Geometry: final body of the model. Coordinates: model frame, mm. A direction names the side the tool comes from. Give positions to 0.01 mm unless a question says otherwise; leave off trailing zeros. Write each loop counter-clockwise with the first axis right and the second up, starting at its lowest first coordinate (ties: lowest second). Pieces come first, ordered by that corner, then holes. Notation, with made-up numbers: (9.5, 86.5) - (27.5, 86.5) arc R19 cw to (27.5, 122.5) - close; hole circle Ø1 at (-33, 45). An arc over 180 degrees is marked (long way). Use CSV: the item, a comma, the result in double quotes. Start each with the question number.
(1) First-contact query: pin 1 Ø4 at (x, y) = (0, 0) entering from +Z. Flat tip, straight axial feed; report the tip coordinate or a pass-through.
(2) Section A-A on z = 3.75. Output: boundary loops of the cut face in (x, y).
(3) Draft query along X for faces 3 (the flat face through (0, 10, 6)), 4 (the flat face through (-10, 0, 6)), 5 (the flat face through (3, 0, 7)), 6 (the cylindrical face through (9.715, 9.699, 6.591)). Return one class per face: released by +X, released by -X, zero draft, split by the parting line, or undercut.
(4) Line query: probe 1 along Y at (x, z) = (0, 5.4); probe 2 along Y at (x, z) = (0, 2); probe 3 along Z at (x, y) = (-3.75, -6.25). Output: solid intervals per line, ascending. Write a range as [from, to].
(5) Section C-C on y = -0.75. Output: boundary loops of the cut face in (x, z).
(6) Section B-B on x = 0. Output: boundary loops of the cut face in (y, z).
(7) Section D-D on z = 7.5. Output: boundary loops of the cut face in (x, y), and give its area (3 significant figures).
(8) Reachability of faces 1 (the flat face through (0, -10, 6)), 2 (the flat face through (-5, 0, 10)) from +Z, -Z, +X, -X, +Y, -Y: full face, straight path, thin tool, end or side. Return the list, or none.
from build123d import *

# Parameters (mm, degrees)
F0_W      = 20
F0_H      = 20
F1_DEPTH  = 13
F2_R      = 1
F3_W      = 10
F3_H      = 11.2
F4_DEPTH  = 6
F5_R      = 2.75
F6_DEPTH  = 3
F8_DEPTH  = 6
F9_R      = 1.5
F10_DEPTH = 4.001


with BuildPart() as f1:
    # F0 (on Top) → F1 (new body)
    with BuildSketch(Plane.XY):
        Rectangle(F0_W, F0_H)
    extrude(amount=F1_DEPTH)

    # F2
    f2_edges = [f1.edges().sort_by_distance(p)[0] for p in [
        (10, -10, 6.5),
        (10, 10, 6.5),
        (-10, 10, 6.5),
        (-10, -10, 6.5),
    ]]
    fillet(f2_edges, radius=F2_R)

    # F3 (on face) → F4 (cut)
    with BuildSketch(Plane.XY.offset(13)):
        Rectangle(F3_W, F3_H)
    extrude(amount=-F4_DEPTH, mode=Mode.SUBTRACT)

    # F5 (on face) → F6 (cut)
    with BuildSketch(Plane.XY.offset(7)):
        Circle(F5_R)
    extrude(amount=-F6_DEPTH, mode=Mode.SUBTRACT)

    # F7 (on face) → F8 (cut)
    with BuildSketch(Plane.XY.offset(13)):
        with BuildLine():
            ThreePointArc((7, 5.6), (5, 7.6), (3, 5.6))
            Line((3, 5.6), (5, 5.6))
            Line((5, 5.6), (5, 3.6))
            ThreePointArc((5, 3.6), (6.4142135624, 4.1857864376), (7, 5.6))
        make_face()
        with BuildLine():
            Line((-5, -5.6), (-5, -3.6))
            ThreePointArc((-5, -3.6), (-6.4142135624, -7.0142135624), (-3, -5.6))
            Line((-3, -5.6), (-5, -5.6))
        make_face()
        with BuildLine():
            ThreePointArc((7, -5.6), (6.4142135624, -4.1857864376), (5, -3.6))
            Line((5, -3.6), (5, -5.6))
            Line((5, -5.6), (3, -5.6))
            ThreePointArc((3, -5.6), (5, -7.6), (7, -5.6))
        make_face()
        with BuildLine():
            Line((-5, 5.6), (-3, 5.6))
            ThreePointArc((-3, 5.6), (-6.4142135624, 7.0142135624), (-5, 3.6))
            Line((-5, 3.6), (-5, 5.6))
        make_face()
    extrude(amount=-F8_DEPTH, mode=Mode.SUBTRACT)

    # F9 (on face) → F10 (cut, through all)
    with BuildSketch(Plane.XY.offset(4)):
        Circle(F9_R)
    extrude(amount=-F10_DEPTH, mode=Mode.SUBTRACT)


solid = f1.part
Check values:
1,pin 1,"stops at z = 4"
2,outline,"(-10, -9) arc R1 ccw to (-9, -10) - (9, -10) arc R1 ccw to (10, -9) - (10, 9) arc R1 ccw to (9, 10) - (-9, 10) arc R1 ccw to (-10, 9) - close; hole circle Ø3 at (0, 0)"
3,face 3,"zero draft"
3,face 4,"released by -X"
3,face 5,"undercut"
3,face 6,"released by +X"
4,probe 1,"y = [-10, -2.75], [2.75, 10]"
4,probe 2,"y = [-10, -1.5], [1.5, 10]"
4,probe 3,"z = [0, 7]"
5,outline,"(-10, 0) - (-1.3, 0) - (-1.3, 4) - (-2.65, 4) - (-2.65, 7) - (-5, 7) - (-5, 13) - (-10, 13) - close; (1.3, 0) - (10, 0) - (10, 13) - (5, 13) - (5, 7) - (2.65, 7) - (2.65, 4) - (1.3, 4) - close"
6,outline,"(-10, 0) - (-1.5, 0) - (-1.5, 4) - (-2.75, 4) - (-2.75, 7) - (-5.6, 7) - (-5.6, 13) - (-10, 13) - close; (1.5, 0) - (10, 0) - (10, 13) - (5.6, 13) - (5.6, 7) - (2.75, 7) - (2.75, 4) - (1.5, 4) - close"
7,outline,"(-10, -9) arc R1 ccw to (-9, -10) - (9, -10) arc R1 ccw to (10, -9) - (10, 9) arc R1 ccw to (9, 10) - (-9, 10) arc R1 ccw to (-10, 9) - close; hole (-5, -3.6) arc R2 ccw (long way) to (-3, -5.6) - (3, -5.6) arc R2 ccw (long way) to (5, -3.6) - (5, 3.6) arc R2 ccw (long way) to (3, 5.6) - (-3, 5.6) arc R2 ccw (long way) to (-5, 3.6) - close"
7,area,"249 mm²"
8,face 1,"+Z, -Z, +X, -X, -Y"
8,face 2,"+Z"
